Could you check a few things on this model? Use its own coordinates, in mm. Give positions to 0.01 mm unless a question says otherwise; leave off trailing zeros. Order: outer loops, then holes, each group sorted by start corner. A loop starts at its lowest first (then second) coordinate and runs counter-clockwise, first axis right, second up. Notation, with made-up numbers: (-19.5, 52) - (-13.5, 52) arc R17 cw to (-13.5, 61) - close; hole circle Ø10 at (73, 84). An arc over 180 degrees is marked (long way). One line per question, with ' | ' between items. Start each with the question number.
1. Imagine slicing it at D-D (x = -18). Please give me the cut outline in (y, z).
2. Imagine slicing it at C-C (z = 10). Please give me the cut outline in (x, y).
3. For P1, Ø16.5, axis at y = -7.46, z = 40.5, coming from the -X side, with a flat end and sliding along its axis, tell me the tip position at first contact or that it passes through.
4. Imagine slicing it at A-A (x = -8.5). Please give me the cut outline in (y, z), and give its area (3 significant figures).
5. Imagine slicing it at B-B (y = -6.5). Please give me the cut outline in (x, z), and give its area (3 significant figures).
6. I need wall thicknesses on probe 1 along Z at (x, y) = (-20, -7); probe 2 along Y at (x, z) = (-16.5, 55); probe 3 along Y at (x, z) = (-1.5, 34.5). Which ranges of each line are inside material? Lowest first, please. Write a range as from..to.
7. If we mould it in two halves opening along Y, with no side actions, what happens to faces 1 (the flat face through (0, -44.934, 38)), 2 (the cylindrical face through (-24.82, 41.31, 37.57)), 3 (the cylindrical face through (-0.401, 6.437, 41.111)), 4 (the flat face through (28.639, 9, 38))? For each: released by +Y, released by -Y, zero draft, split by the parting line, or undercut.
```python
from build123d import *

# Parameters (mm, degrees)
F1_DEPTH = 76.2
F2_R     = 8.443536
F3_DEPTH = 76.201
F4_R     = 13.907635
F5_DEPTH = 57.279376


with BuildPart() as f1:
    # F0 (on Top) → F1 (new body)
    with BuildSketch(Plane.XY):
        with BuildLine():
            Line((-28.639188, 32.2339), (-28.639188, -44.9339))
            Line((-28.639188, -44.9339), (28.639188, -44.9339))
            Line((28.639188, -44.9339), (28.639188, 44.9339))
            Line((28.639188, 44.9339), (-15.939188, 44.9339))
            ThreePointArc((-15.939188, 44.9339), (-24.919444, 41.214156), (-28.639188, 32.2339))
        make_face()
    extrude(amount=F1_DEPTH)

    # F2 (on face) → F3 (cut, through all)
    with BuildSketch(Plane.XY.offset(76.2)):
        with Locations((-13.24562, -18.163707)):
            Circle(F2_R)
    extrude(amount=-F3_DEPTH, mode=Mode.SUBTRACT)

    # F4 (on face) → F5 (cut, through all)
    with BuildSketch(Plane(origin=(-28.639188, 0, 0), x_dir=(0, -1, 0), z_dir=(-1, 0, 0))):
        with Locations((7.457322, 40.499449)):
            Circle(F4_R)
    extrude(amount=-F5_DEPTH, mode=Mode.SUBTRACT)


solid = f1.part
```
Results found:
1) outline: (-44.93, 0) - (-25.14, 0) - (-25.14, 76.2) - (-44.93, 76.2) - close; (-11.19, 0) - (44.77, 0) - (44.77, 76.2) - (-11.19, 76.2) - (-11.19, 53.9) arc R13.91 cw (long way) to (-11.19, 27.1) - close
2) outline: (-28.64, -44.93) - (28.64, -44.93) - (28.64, 44.93) - (-15.94, 44.93) arc R12.7 ccw to (-28.64, 32.23) - close; hole circle Ø16.89 at (-13.25, -18.16)
3) P1: passes through
4) outline: (-44.93, 0) - (-25.15, 0) - (-25.15, 76.2) - (-44.93, 76.2) - close; (-11.18, 0) - (44.93, 0) - (44.93, 76.2) - (-11.18, 76.2) - (-11.18, 53.9) arc R13.91 cw (long way) to (-11.18, 27.1) - close | area: 5,380 mm2
5) outline: (-28.64, 0) - (28.64, 0) - (28.64, 26.62) - (-28.64, 26.62) - close; (-28.64, 54.37) - (28.64, 54.37) - (28.64, 76.2) - (-28.64, 76.2) - close | area: 2,780 mm2
6) probe 1: z = 0..26.6, 54.4..76.2 | probe 2: y = -44.93..-25.95, -10.37..44.92 | probe 3: y = -44.93..-20, 5.09..44.93
7) face 1: released by -Y | face 2: released by +Y | face 3: undercut | face 4: zero draft
